Build history of the part. All positions in model axes, mm. A direction names the side the tool comes from. Coordinates: 2 decimals unless noted, no trailing zeros. Loops run counter-clockwise (first coordinate to the right, second up) from the corner with the lowest first, then second, coordinate; pieces in that order, holes last.
Item 1: Cut at C-C (y = 0). List the corners of the cut face in (x, z), and give its area (3 significant figures).
Item 2: Flat gauge pins, fed straight in: pin 1 (10 mm diameter, centred on x = 1, y = -49.5, fed in from +Z); pin 2 (2 mm diameter, centred on y = -38.5, z = 2, fed in from -X). Where does each tip first touch, or does it go through?
Item 3: Cut at A-A (x = -13). List the corners of the cut face in (y, z), and give its area (3 significant figures).
Item 4: 3-axis set-ups, long thin cutter, end or side, ignore diameter. For faces 4 (the face through (3.57, -19, 2.03)), 5 (the face through (0, 12.5, 2)), 6 (the face through (0, 17.5, 2)), 7 (the face through (10, -37, 2)), 8 (the face through (0, -13, 4)): which of +Z, -Z, +X, -X, +Y, -Y reach the whole face in a straight line?
Item 5: Drill centre lines: line 1 along Y through (x, z) = (0, 1.25); line 2 along Y through (x, z) = (-1, 0.95); line 3 along Y through (x, z) = (-12.5, 1.05). Where is each one in solid material? Low to high.
Item 6: Cut at D-D (y = -47.5). List the corners of the cut face in (x, z), and give its area (3 significant figures).
Item 7: Mould opens along X. For faces 1 (the face through (-0.488, -57.052, 1.972)), 2 (the face through (-1.45, -61.97, 1.97)), 3 (the face through (11.43, -19, 2.03)) say: released by +X, released by -X, zero draft, split by the parting line, or undercut.
from build123d import *

# Parameters (mm, degrees)
F1_DEPTH = 4
F2_R     = 4.99999


# Not quite as in the source:
# - a fillet or chamfer is up to 0.001 mm smaller than in the source, because OpenCascade refuses the exact size


with BuildPart() as f1:
    # F0 (on Top) → F1 (new body)
    with BuildSketch(Plane.XY):
        with BuildLine():
            ThreePointArc((5, -52.0760789514), (-0.6060621786, -57.039211897), (-4.8530754543, -50.8728920851))
            Line((-4.8530754543, -50.8728920851), (-9.7061509086, -49.6697052189))
            ThreePointArc((-9.7061509086, -49.6697052189), (-1.2121243571, -62.0023448426), (10, -52.0760789514))
            Line((10, -52.0760789514), (10, -20.8603814244))
            Line((10, -20.8603814244), (10, -17.5000000745))
            Line((10, -17.5000000745), (15, -17.5000000745))
            ThreePointArc((15, -17.5000000745), (32.5000000745, 0), (15, 17.5000000745))
            Line((15, 17.5000000745), (0, 17.5000000745))
            Line((0, 17.5000000745), (-15, 17.5000000745))
            ThreePointArc((-15, 17.5000000745), (-32.5000000745, 0), (-15, -17.5000000745))
            Line((-15, -17.5000000745), (0, -17.5000000745))
            Line((0, -17.5000000745), (5, -17.5000000745))
            Line((5, -17.5000000745), (5, -18.7957836315))
            Line((5, -18.7957836315), (5, -43.4158249135))
            Line((5, -43.4158249135), (5, -52.0760789514))
        make_face()
        with BuildLine():
            ThreePointArc((-15, -12.5), (-27.5, 0), (-15, 12.5))
            Line((-15, 12.5), (0, 12.5))
            Line((0, 12.5), (15, 12.5))
            ThreePointArc((15, 12.5), (27.5, 0), (15, -12.5))
            Line((15, -12.5), (0, -12.5))
            Line((0, -12.5), (-15, -12.5))
        make_face(mode=Mode.SUBTRACT)
    extrude(amount=F1_DEPTH)

    # F2 (radius 5 in the source; OpenCascade refuses exactly that, so slightly less here)
    f2_edges = [f1.edges().sort_by_distance(p)[0] for p in [
        (5, -17.5, 2),
        (10, -17.5, 2),
    ]]
    fillet(f2_edges, radius=F2_R)


solid = f1.part
Filled sheet:
1. outline: (-32.5, 0) - (-27.5, 0) - (-27.5, 4) - (-32.5, 4) - close; (27.5, 0) - (32.5, 0) - (32.5, 4) - (27.5, 4) - close
1. area: 40.0 mm2
2. pin 1: stops at z = 4
2. pin 2: stops at x = 5
3. outline: (-17.5, 0) - (-12.5, 0) - (-12.5, 4) - (-17.5, 4) - close; (12.5, 0) - (17.5, 0) - (17.5, 4) - (12.5, 4) - close
3. area: 40.0 mm2
4. face 4: +Z, -Z, -X
4. face 5: +Z, -Z
4. face 6: +Z, -Z, +X, -X, +Y
4. face 7: +Z, -Z, +X, -Y
4. face 8: +Z, +X, -X, +Y, -Y
5. line 1: y = -62.08 to -57.08, -17.5 to -12.5, 12.5 to 17.5
5. line 2: y = -62.03 to -56.98, -17.5 to -12.5, 12.5 to 17.5
5. line 3: y = -17.5 to -12.5, 12.5 to 17.5
6. outline: (5, 0) - (10, 0) - (10, 4) - (5, 4) - close
6. area: 20.0 mm2
7. face 1: undercut
7. face 2: split by the parting line
7. face 3: released by +X
